Verification items for the finished model (mm, model axes). Face numbers are marked on the shaded views. A direction names the side the tool comes from. Coordinates: 2 decimals unless noted, no trailing zeros. Write each loop counter-clockwise with the first axis right and the second up, starting at its lowest first coordinate (ties: lowest second). Pieces come first, ordered by that corner, then holes. Notation, with made-up numbers: (-11, 15) -> (25, 15) arc R10 cw to (25, 26) -> close; hole circle Ø1 at (18, 72.5). An arc over 180 degrees is marked (long way). Write item = value, one per line. Start each with the question number.
(1) Section check D-D (y = 23.5). Record the cut outline in (x, z).
(2) Section check A-A (y = 16). Record the cut outline in (x, z).
(3) Gauge pin test, flat ends, axial feed: pin 1 Ø1.5 at (x, y) = (1.5, 43.5) entering from -Z; pin 2 Ø3 at (x, y) = (2, 28) entering from -Z; pin 3 Ø2.5 at (x, z) = (3.5, 37) entering from +Y. Record the tip position at first contact, or that the pin passes through.
(4) Section check B-B (z = 20). Record the cut outline in (x, y).
(5) Material ranges on probe 1 along Y at (x, z) = (2.65, 4); probe 2 along Y at (x, z) = (1.75, 12); probe 3 along Y at (x, z) = (0.9, 23.5), recorded low to high. Write a range as [from, to].
(6) Section check C-C (x = 0.8). State how many separate pieces and enclosed holes the cut face has, plus the area to 3 significant figures.
(7) Mould release check, pull along Z, two halves, no side actions. Record for the marked faces 1, 2, 3 and 4: released by +Z, released by -Z, zero draft, split by the parting line, or undercut.
(8) Set-up check for the marked faces 5, 6, 7 and 8: record each of +Z, -Z, +X, -X, +Y, -Y from which the full face is reachable in a straight line by a thin tool's end or side.
```python
from build123d import *

# Parameters (mm, degrees)
SKETCH_1_R      = 5.1
EXTRUDE_1_DEPTH = 5


with BuildPart() as part:
    # 草图1 → 凸台-拉伸1 (new body)
    with BuildSketch(Plane(origin=(0, 0, 0), x_dir=(0, 0, -1), z_dir=(1, 0, 0))):
        Polygon((-30, 40), (-40, 40), (-40, 30), (-35, 30), (-35, 10), (-40, 10), (-40, 0), (0, 0), (0, 10), (-5, 10), (-5, 30), (0, 30), (0, 40), (-10, 40), (-10, 45), (-30, 45), align=None)
        with Locations((-20, 16)):
            Circle(SKETCH_1_R, mode=Mode.SUBTRACT)
        with BuildLine():
            ThreePointArc((-24.298590679, 24.751263804), (-26.780876657, 23.005869808), (-28.606339093, 20.58185851))
            ThreePointArc((-28.606339093, 20.58185851), (-27.883996425, 18.21474612), (-25.516884034, 18.937088789))
            ThreePointArc((-25.516884034, 18.937088789), (-24.346715806, 20.490942184), (-22.755506846, 21.60978449))
            ThreePointArc((-22.755506846, 21.60978449), (-21.956309105, 23.952066064), (-24.298590679, 24.751263804))
        make_face(mode=Mode.SUBTRACT)
        with BuildLine():
            ThreePointArc((-11.248736196, 20.298590679), (-12.994130192, 22.780876657), (-15.41814149, 24.606339093))
            ThreePointArc((-15.41814149, 24.606339093), (-17.78525388, 23.883996425), (-17.062911211, 21.516884034))
            ThreePointArc((-17.062911211, 21.516884034), (-15.509057816, 20.346715806), (-14.39021551, 18.755506846))
            ThreePointArc((-14.39021551, 18.755506846), (-12.047933936, 17.956309105), (-11.248736196, 20.298590679))
        make_face(mode=Mode.SUBTRACT)
        with BuildLine():
            ThreePointArc((-15.701409321, 7.248736196), (-13.219123343, 8.994130192), (-11.393660907, 11.41814149))
            ThreePointArc((-11.393660907, 11.41814149), (-12.116003575, 13.78525388), (-14.483115966, 13.062911211))
            ThreePointArc((-14.483115966, 13.062911211), (-15.653284194, 11.509057816), (-17.244493154, 10.39021551))
            ThreePointArc((-17.244493154, 10.39021551), (-18.043690895, 8.047933936), (-15.701409321, 7.248736196))
        make_face(mode=Mode.SUBTRACT)
        with BuildLine():
            ThreePointArc((-28.751263804, 11.701409321), (-27.005869808, 9.219123343), (-24.58185851, 7.393660907))
            ThreePointArc((-24.58185851, 7.393660907), (-22.21474612, 8.116003575), (-22.937088789, 10.483115966))
            ThreePointArc((-22.937088789, 10.483115966), (-24.490942184, 11.653284194), (-25.60978449, 13.244493154))
            ThreePointArc((-25.60978449, 13.244493154), (-27.952066064, 14.043690895), (-28.751263804, 11.701409321))
        make_face(mode=Mode.SUBTRACT)
    extrude(amount=EXTRUDE_1_DEPTH)


solid = part.part
```
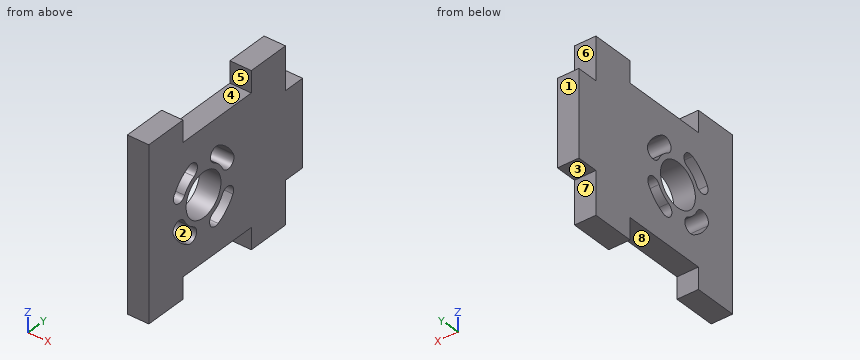
Response:
q1.outline = (0, 5) -> (5, 5) -> (5, 13.77) -> (0, 13.77) -> close; (0, 17.93) -> (5, 17.93) -> (5, 21.81) -> (0, 21.81) -> close; (0, 26.23) -> (5, 26.23) -> (5, 35) -> (0, 35) -> close
q2.outline = (0, 5) -> (5, 5) -> (5, 14.9) -> (0, 14.9) -> close; (0, 25.1) -> (5, 25.1) -> (5, 35) -> (0, 35) -> close
q3.pin_1 = 10
q3.pin_2 = 5
q3.pin_3 = 40
q4.outline = (0, 0) -> (5, 0) -> (5, 10.9) -> (0, 10.9) -> close; (0, 21.1) -> (5, 21.1) -> (5, 45) -> (0, 45) -> close
q5.probe_1 = [0, 10], [30, 40]
q5.probe_2 = [0, 10.43], [13.72, 17.98], [21.57, 45]
q5.probe_3 = [0, 7.21], [10.82, 12.29], [19.71, 21.18], [24.93, 45]
q6.separate_pieces = 1
q6.enclosed_holes = 5
q6.area = 1,310 mm2
q7.face_1 = zero draft
q7.face_2 = undercut
q7.face_3 = released by -Z
q7.face_4 = released by +Z
q8.face_5 = +Z, +X, -X
q8.face_6 = +Z, +X, -X, +Y
q8.face_7 = -Z, +X, -X, +Y
q8.face_8 = -Z, +X, -X
